```python
from build123d import *

# Parameters (mm, degrees)
F1_DEPTH = 215.9
F2_W     = 50.8
F2_H     = 9.525
F3_DEPTH = 50.8
F5_DEPTH = 50.801


with BuildPart() as f1:
    # F0 (on Front) → F1 (new body)
    with BuildSketch(Plane.XZ):
        with BuildLine():
            Line((9.525, 50.8), (0, 50.8))
            Line((0, 50.8), (0, 6.35))
            ThreePointArc((0, 6.35), (1.859872, 1.859872), (6.35, 0))
            Line((6.35, 0), (76.2, 0))
            Line((76.2, 0), (76.2, 9.525))
            Line((76.2, 9.525), (15.875, 9.525))
            ThreePointArc((15.875, 9.525), (11.384872, 11.384872), (9.525, 15.875))
            Line((9.525, 15.875), (9.525, 50.8))
        make_face()
    extrude(amount=F1_DEPTH)

    # F2 (on face) → F3 (join)
    with BuildSketch(Plane(origin=(0, 0, 0), x_dir=(-1, 0, 0), z_dir=(0, 1, 0))):
        with Locations((-50.8, 4.7625)):
            Rectangle(F2_W, F2_H)
    extrude(amount=F3_DEPTH)

    # F4 (on face) → F5 (cut, through all)
    with BuildSketch(Plane(origin=(0, 0, 0), x_dir=(1, 0, 0), z_dir=(0, 0, -1))):
        with BuildLine():
            Line((44.45, 25.4), (44.45, -14.401477))
            ThreePointArc((44.45, -14.401477), (50.8, -38.1), (57.15, -14.401477))
            Line((57.15, -14.401477), (57.15, 25.4))
            ThreePointArc((57.15, 25.4), (50.8, 31.75), (44.45, 25.4))
        make_face()
    extrude(amount=-F5_DEPTH, mode=Mode.SUBTRACT)


solid = f1.part
```
The model under review builds one solid part; all positions refer to its coordinate system, in mm. A direction names the side the tool comes from. Coordinates: 2 decimals unless noted, no trailing zeros. Order: outer loops, then holes, each group sorted by start corner. A loop starts at its lowest first (then second) coordinate and runs counter-clockwise, first axis right, second up. Notation, with made-up numbers: (10, 8) -> (24, 8) arc R18 cw to (24, 28) -> close; hole circle Ø9 at (38.5, 21.5). An arc over 180 degrees is marked (long way). Answer in a Markdown table with one row per item. Add a question column.
Item 1: Mouldability with a two-part tool opening along X and no side actions: class faces 6 (the cylindrical face through (11.43, -106.44, 11.34)), 7 (the flat face through (57.15, -5, 5)), 8 (the flat face through (27, -215.9, 9)), 9 (the flat face through (25.4, 25, 5)) as +X half, -X half, draft (parallel to the pull), parting line (faces both ways), or undercut.
Item 2: We need section A-A on y = 25.4. Write out the cut boundary in (x, z) (3 decimals), plus the area to 3 significant figures.
Item 3: We need section C-C on y = -102.5. Write out the cut boundary in (x, z) (3 decimals).
Item 4: Clearance check with flat-ended pins moving along their axes: pin 1 (20.5 mm diameter, centred on x = 8.5, z = 29.5, fed in from +Y); pin 2 (18 mm diameter, centred on x = 33.5, y = -115.5, fed in from +Z) (3 decimals); pin 3 (4 mm diameter, centred on y = -21.5, z = 34.5, fed in from +X) (3 decimals). State where each tip first meets the part, or that it passes through.
Item 5: To check wall thickness, follow probe 1 along X at (y, z) = (25.4, 5); probe 2 along Y at (x, z) = (50.8, 4.5); probe 3 along Z at (x, y) = (18, -10) (3 decimals). State the ranges of each line that lie inside material, in increasing order.
Item 6: Machinability: for faces 1 (the flat face through (5, -106, 50.8)), 2 (the flat face through (51, 50.8, 5)), 3 (the flat face through (44.45, -6, 5)), 4 (the flat face through (9.525, -106, 33)), 5 (the flat face through (7, 0, 20)), which of the approach directions +Z, -Z, +X, -X, +Y, -Y give a long, thin tool a straight path to every point of the face, cutting with its end or side? Answer none if there is none.
Item 7: We need section B-B on x = 50.8. Write out the cut boundary in (y, z) (3 decimals), plus the area to 4 significant figures.
Item 8: We need section D-D on z = 33. Write out the cut boundary in (x, y) (3 decimals), plus the area to 3 significant figures.
Final values:
| question | item | result |
|---|---|---|
| 1 | face 6 | +X half |
| 1 | face 7 | undercut |
| 1 | face 8 | draft |
| 1 | face 9 | -X half |
| 2 | outline | (25.4, 0) -> (38.1, 0) -> (38.1, 9.525) -> (25.4, 9.525) -> close; (63.5, 0) -> (76.2, 0) -> (76.2, 9.525) -> (63.5, 9.525) -> close |
| 2 | area | 242 mm2 |
| 3 | outline | (0, 6.35) arc R6.35 ccw to (6.35, 0) -> (76.2, 0) -> (76.2, 9.525) -> (15.875, 9.525) arc R6.35 cw to (9.525, 15.875) -> (9.525, 50.8) -> (0, 50.8) -> close |
| 4 | pin 1 | stops at y = 0 |
| 4 | pin 2 | stops at z = 9.525 |
| 4 | pin 3 | stops at x = 9.525 |
| 5 | probe 1 | x = 25.4 to 38.1, 63.5 to 76.2 |
| 5 | probe 2 | y = -215.9 to -31.75, 38.1 to 50.8 |
| 5 | probe 3 | z = 0 to 9.525 |
| 6 | face 1 | +Z, +X, -X, +Y, -Y |
| 6 | face 2 | +Z, -Z, +X, -X, +Y |
| 6 | face 3 | +Z, -Z |
| 6 | face 4 | +Z, +X, +Y, -Y |
| 6 | face 5 | +Z, -Z, -X, +Y |
| 7 | outline | (-215.9, 0) -> (-31.75, 0) -> (-31.75, 9.525) -> (-215.9, 9.525) -> close; (38.1, 0) -> (50.8, 0) -> (50.8, 9.525) -> (38.1, 9.525) -> close |
| 7 | area | 1,875 mm2 |
| 8 | outline | (0, -215.9) -> (9.525, -215.9) -> (9.525, 0) -> (0, 0) -> close |
| 8 | area | 2,060 mm2 |
